The drawing under review shows one solid part. Ordinate dimensions are in mm from its lowest x, y, z. Round coordinates to 2 decimals unless told otherwise and drop trailing zeros. Loops run counter-clockwise (first coordinate to the right, second up) from the corner with the lowest first, then second, coordinate; pieces in that order, holes last. Notation, with made-up numbers: M 15,16 L 54,16 A27 ccw 54,34 Z; hole C 60,21 d1. An arc over 180 degrees is marked long. Use a Markdown table: item, result.
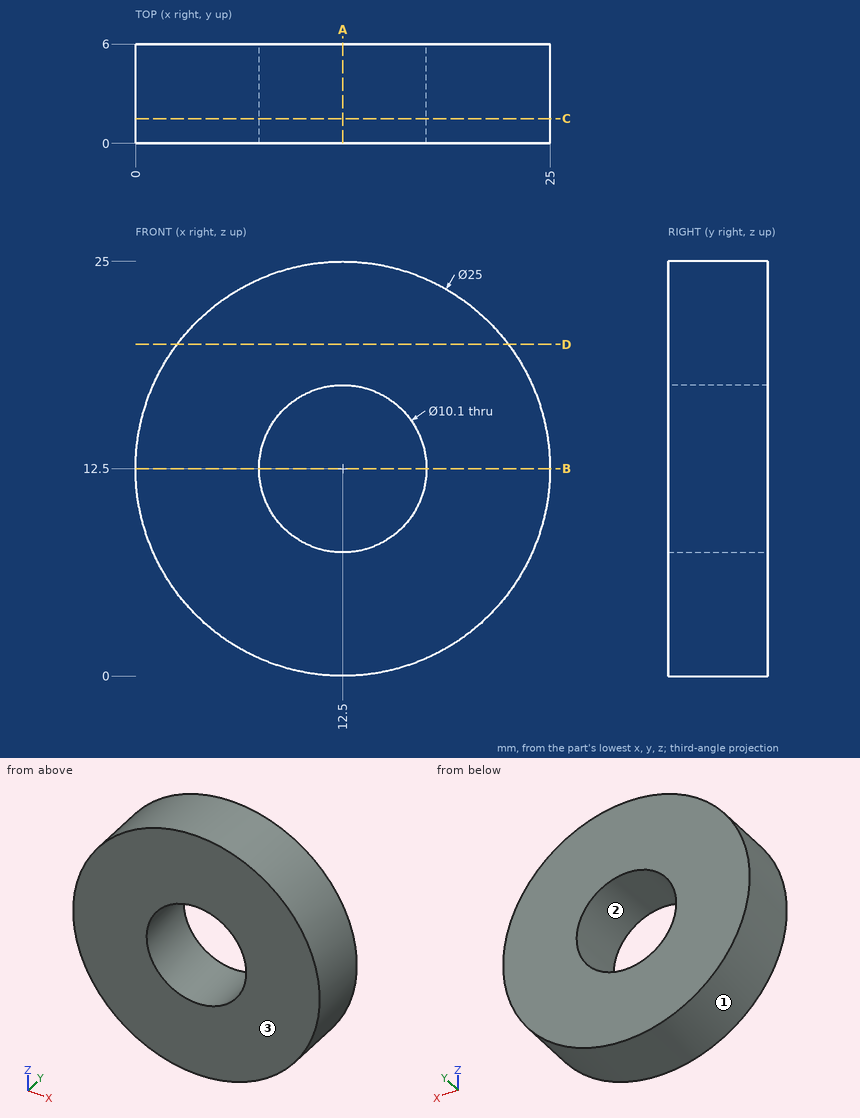
1. Take a section at A-A on x = 12.5. Give the boundary of the cut face in (y, z).
Check values:
| item | result |
|---|---|
| outline | M 0,0 L 6,0 L 6,7.45 L 0,7.45 Z; M 0,17.55 L 6,17.55 L 6,25 L 0,25 Z |
2. Wall thickness on line 1 along X through (y, z) = (3.3, 12.5); line 2 along Z through (x, y) = (16, 2.35); line 3 along X through (y, z) = (2.1, 6.5): over which ranges is each line inside the solid? List them lowest first. Write a range as from..to.
Check values:
| item | result |
|---|---|
| line 1 | x = 0..7.45, 17.55..25 |
| line 2 | z = 0.5..8.86, 16.14..24.5 |
| line 3 | x = 1.53..23.47 |
3. Take a section at B-B on z = 12.5. Give the boundary of the cut face in (x, y), and give its area (3 significant figures).
Check values:
| item | result |
|---|---|
| outline | M 0,0 L 7.45,0 L 7.45,6 L 0,6 Z; M 17.55,0 L 25,0 L 25,6 L 17.55,6 Z |
| area | 89.4 mm² |
4. Take a section at C-C on y = 1.5. Give the boundary of the cut face in (x, z), and give its area (3 significant figures).
Check values:
| item | result |
|---|---|
| outline | C 12.5,12.5 d25; hole C 12.5,12.5 d10.1 |
| area | 411 mm² |
5. The part is to be moulded in two halves that separate along Z. For the marked faces 1, 2 and 3, say which applies: pulls with the +Z half, pulls with the -Z half, needs draft (parallel to the pull), parting line crosses it, or undercut.
Check values:
| item | result |
|---|---|
| face 1 | parting line crosses it |
| face 2 | undercut |
| face 3 | needs draft |
6. Insertion check: pin 1 (1.5 mm diameter, centred on y = 2, z = 15.5, fed in from +X). The pin has a flat end and moves straight along its axis. Give the tip position at first contact, or say it passes through.
Check values:
| item | result |
|---|---|
| pin 1 | stops at x = 24.8 |
7. Take a section at D-D on z = 20. Give the boundary of the cut face in (x, y), and give its area (3 significant figures).
Check values:
| item | result |
|---|---|
| outline | M 2.5,0 L 22.5,0 L 22.5,6 L 2.5,6 Z |
| area | 120 mm² |
